Geometry: final body of the model. Coordinates: model frame, mm. Face numbers are marked on the shaded views. Round coordinates to 2 decimals unless told otherwise and drop trailing zeros. Write each loop counter-clockwise with the first axis right and the second up, starting at its lowest first coordinate (ties: lowest second). Pieces come first, ordered by that corner, then holes. Notation, with made-up numbers: (51.25, 10.5) -> (103.25, 10.5) arc R24 ccw to (103.25, 46.5) -> close; hole circle Ø8 at (-23.5, 51.5). An arc over 180 degrees is marked (long way). One line per item, written item: value. Start each with the question number.
from build123d import *

# Parameters (mm, degrees)
SKETCH_1_R      = 30
SKETCH_1_R_2    = 23
EXTRUDE_1_DEPTH = 21
SKETCH_2_R      = 23
SKETCH_2_R_2    = 4.1
SKETCH_2_R_3    = 1.55
EXTRUDE_2_DEPTH = 4


with BuildPart() as part:
    # 草图1 → 凸台-拉伸1 (new body)
    with BuildSketch(Plane(origin=(0, 0, 0), x_dir=(1, 0, 0), z_dir=(0, 1, 0))):
        with Locations(Location((0, 0, 0), (0, 0, 90))):
            Circle(SKETCH_1_R)
        with Locations(Location((0, 0, 0), (0, 0, 90))):
            Circle(SKETCH_1_R_2, mode=Mode.SUBTRACT)
    extrude(amount=EXTRUDE_1_DEPTH)

    # 草图2 → 凸台-拉伸2 (add)
    with BuildSketch(Plane.XZ):
        with Locations(Location((0, 0, 0), (0, 0, 270))):
            Circle(SKETCH_2_R)
        with Locations(Location((0, 0, 0), (0, 0, 270))):
            Circle(SKETCH_2_R_2, mode=Mode.SUBTRACT)
        with Locations(Location((6, 0, 0), (0, 0, 270))):
            Circle(SKETCH_2_R_3, mode=Mode.SUBTRACT)
        with Locations(Location((-6, 0, 0), (0, 0, 270))):
            Circle(SKETCH_2_R_3, mode=Mode.SUBTRACT)
        with Locations(Location((0, 6.5, 0), (0, 0, 270))):
            Circle(SKETCH_2_R_3, mode=Mode.SUBTRACT)
        with Locations(Location((0, -6.5, 0), (0, 0, 270))):
            Circle(SKETCH_2_R_3, mode=Mode.SUBTRACT)
        with BuildLine():
            ThreePointArc((13.744660155, 13.324975875), (0.2967616, 19.141123201), (-13.324975875, 13.744660155))
            ThreePointArc((-13.324975875, 13.744660155), (-13.412668503, 8.088485652), (-7.756494001, 8.000793024))
            ThreePointArc((-7.756494001, 8.000793024), (0.172745496, 11.142084508), (8.000793024, 7.756494001))
            ThreePointArc((8.000793024, 7.756494001), (13.656967527, 7.668801373), (13.744660155, 13.324975875))
        make_face(mode=Mode.SUBTRACT)
        with BuildLine():
            ThreePointArc((13.744660155, -13.324975875), (0.2967616, -19.141123201), (-13.324975875, -13.744660155))
            ThreePointArc((-13.324975875, -13.744660155), (-13.412668503, -8.088485652), (-7.756494001, -8.000793024))
            ThreePointArc((-7.756494001, -8.000793024), (0.172745496, -11.142084508), (8.000793024, -7.756494001))
            ThreePointArc((8.000793024, -7.756494001), (13.656967527, -7.668801373), (13.744660155, -13.324975875))
        make_face(mode=Mode.SUBTRACT)
    extrude(amount=-EXTRUDE_2_DEPTH)


solid = part.part
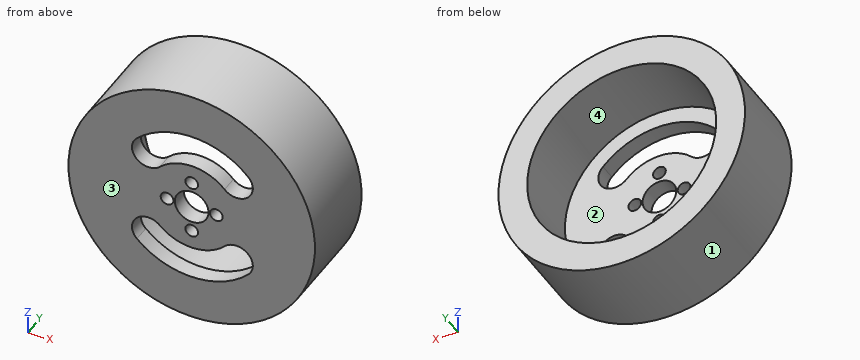
(1) Section query C-C (z = -16.5). Output: boundary loops of the cut face in (x, y), and give its area (3 significant figures).
(2) Section query D-D (y = 15). Output: boundary loops of the cut face in (x, z).
(3) Line query: probe 1 along X at (y, z) = (1.5, 0); probe 2 along X at (y, z) = (16, 0); probe 3 along Y at (x, z) = (16, -1). Output: solid intervals per line, ascending.
(4) Section query B-B (z = 0). Output: boundary loops of the cut face in (x, y).
(5) Pin query (flat end, axial travel): pin 1 (1 mm diameter, centred on y = 7.5, z = 9.5, fed in from +X); pin 2 (12 mm diameter, centred on y = 4.5, z = -1.5, fed in from -X); pin 3 (2 mm diameter, centred on y = 15, z = 24, fed in from +X); pin 4 (1 mm diameter, centred on x = 23, z = -3.5, fed in from -Y). Return the tip coordinate at first contact, or that it passes through.
(6) Section query A-A (x = 0). Output: boundary loops of the cut face in (y, z).
(7) Pull-direction query (X, two-part tool) for the marked faces 1, 2, 3 and 4; classes: pulls with the +X half, pulls with the -X half, needs draft (parallel to the pull), parting line crosses it, or undercut.
Results list:
1. outline: (-25.05, 0) -> (-9.71, 0) -> (-9.71, 4) -> (-16.02, 4) -> (-16.02, 21) -> (-25.05, 21) -> close; (9.71, 0) -> (25.05, 0) -> (25.05, 21) -> (16.02, 21) -> (16.02, 4) -> (9.71, 4) -> close
1. area: 430 mm^2
2. outline: circle Ø60 at (0, 0); hole circle Ø46 at (0, 0)
3. probe 1: x = -30 to -7.55, -4.45 to -4.1, 4.1 to 4.45, 7.55 to 30
3. probe 2: x = -30 to -23, 23 to 30
3. probe 3: y = 0 to 4
4. outline: (-30, 0) -> (-7.55, 0) -> (-7.55, 4) -> (-23, 4) -> (-23, 21) -> (-30, 21) -> close; (-4.45, 0) -> (-4.1, 0) -> (-4.1, 4) -> (-4.45, 4) -> close; (4.1, 0) -> (4.45, 0) -> (4.45, 4) -> (4.1, 4) -> close; (7.55, 0) -> (30, 0) -> (30, 21) -> (23, 21) -> (23, 4) -> (7.55, 4) -> close
5. pin 1: stops at x = 28.62
5. pin 2: stops at x = -30
5. pin 3: stops at x = 19.26
5. pin 4: stops at y = 0
6. outline: (0, -30) -> (21, -30) -> (21, -23) -> (4, -23) -> (4, -19.14) -> (0, -19.14) -> close; (0, -11.14) -> (4, -11.14) -> (4, -8.05) -> (0, -8.05) -> close; (0, -4.95) -> (4, -4.95) -> (4, -4.1) -> (0, -4.1) -> close; (0, 4.1) -> (4, 4.1) -> (4, 4.95) -> (0, 4.95) -> close; (0, 8.05) -> (4, 8.05) -> (4, 11.14) -> (0, 11.14) -> close; (0, 19.14) -> (4, 19.14) -> (4, 23) -> (21, 23) -> (21, 30) -> (0, 30) -> close
7. face 1: parting line crosses it
7. face 2: undercut
7. face 3: needs draft
7. face 4: undercut
